Part model, mm, in its own coordinate system. A direction names the side the tool comes from. Coordinates: 2 decimals unless noted, no trailing zeros. Write each loop counter-clockwise with the first axis right and the second up, starting at its lowest first coordinate (ties: lowest second). Pieces come first, ordered by that corner, then holes. Notation, with made-up numbers: (3, 1.25) -> (59, 1.25) arc R12 cw to (59, 21.25) -> close; hole circle Ø5 at (41, -30). An arc over 180 degrees is marked (long way). Write item = value, one per line. Start each with the question number.
Q1. Tool access for faces 1 (the flat face through (-354.878, 1611, 66)), 2 (the cylindrical face through (-511.78, 1605.4, 68.03)): list every direction of +Z, -Z, +X, -X, +Y, -Y with a clear straight run to the whole face (end or side of a thin tool).
Q2. Probe line 1 (X direction, y = 1655.5, z = 19.5). List the from-to ranges inside material, lowest first.
Q3. Pin check, flat tip, straight feed: P1, Ø14, axis at y = 1808, z = -108.5, coming from the +X side. Stop position of the tip, or through.
Q4. Band-saw the part on A-A, the plane x = -448. List the corners of the cut face in (y, z).
from build123d import *

# Parameters (mm, degrees)
SWEEP1_PROFILE_R = 6.35


with BuildPart() as part:
    # Sweep1: sweep along a curve in space
    with BuildLine() as sweep1_path:
        Line((-635.040454363, 1805.032599319, -106.306821176), (-673.140454363, 1805.032599319, -106.306821176))
        ThreePointArc((-673.140454363, 1805.032599319, -106.306821176), (-691.100966605, 1799.480226411, -101.355343296), (-698.540454363, 1786.075612435, -89.401418245))
        Line((-698.540454363, 1786.075612435, -89.401418245), (-698.540454363, 1630.459986884, 49.373001358))
        ThreePointArc((-673.140454363, 1611.503, 66.278404289), (-691.100966605, 1617.055372908, 61.326926409), (-698.540454363, 1630.459986884, 49.373001358))
        Line((-354.878454363, 1611.503, 66.278404289), (-673.140454363, 1611.503, 66.278404289))
    # Sweep1 profile (on start of the path) → Sweep1 (sweep)
    with BuildSketch(Plane(origin=(-635.040454363, 1805.032599319, -106.306821176), x_dir=(0, 0, -1), z_dir=(-1, 0, 0))):
        Circle(SWEEP1_PROFILE_R)
    sweep(path=sweep1_path.line)


solid = part.part
Ans:
q1.face_1 = +Z, -Z, +X, +Y, -Y
q1.face_2 = +X
q2.line_1 = -701.48 to -695.6
q3.P1 = -635.04
q4.outline = circle Ø12.7 at (1611.5, 66.28)
